Source: three-view drawing plus pictorial views. Frame: mm from the lowest corner of the part. A direction names the side the tool comes from. Coordinates: 2 decimals unless noted, no trailing zeros. Order: outer loops, then holes, each group sorted by start corner. A loop starts at its lowest first (then second) coordinate and runs counter-clockwise, first axis right, second up. Notation, with made-up numbers: (38, 13.5) -> (81, 13.5) arc R16 cw to (81, 20.5) -> close; hole circle Ø4 at (-38.5, 83.25). An arc over 180 degrees is marked (long way). One line per question, with ' | ' between items.
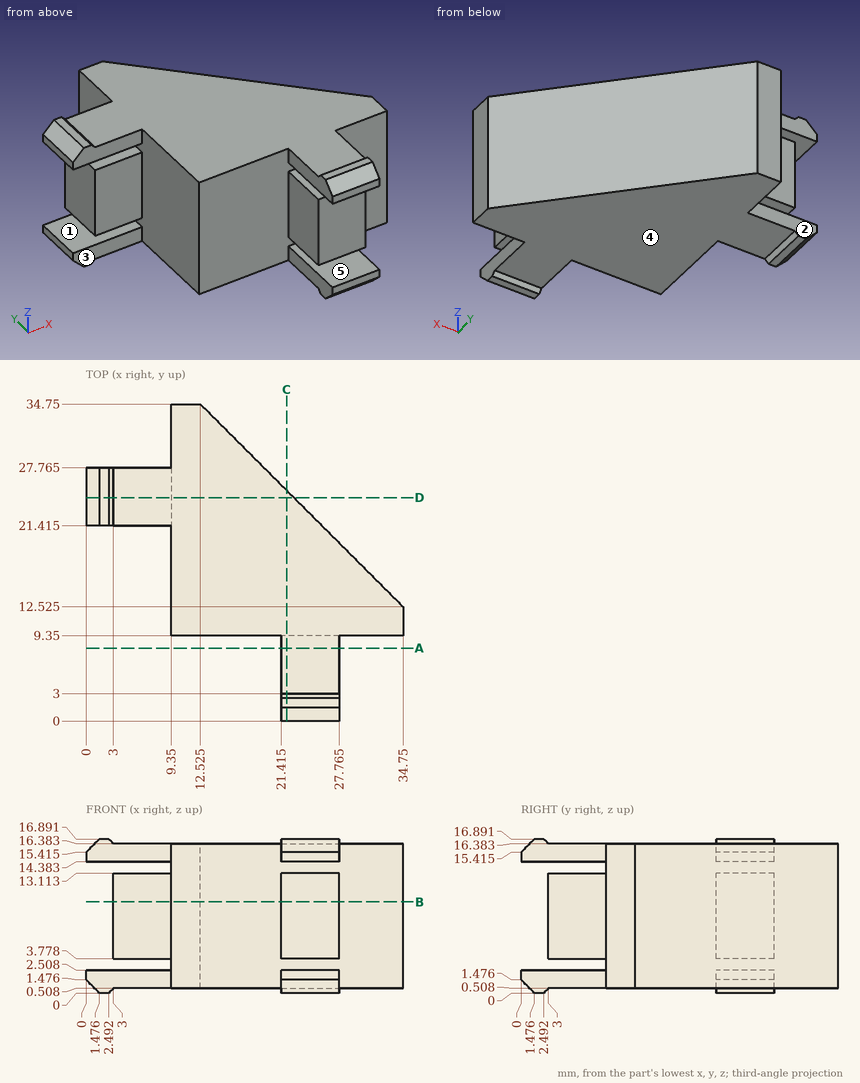
1. Access query for the marked faces 1, 2, 3, 4 and 5. Directions: +Z, -Z, +X, -X, +Y, -Y. A direction counts if a zero-diameter tool reaches every point of the face in a straight line with its end or side. Return the directions, or none.
Recorded:
face 1: -X, +Y, -Y | face 2: +Z, -Z, -X, +Y | face 3: +Z, -Z, -X, -Y | face 4: -Z, +X, +Y | face 5: +X, -X, -Y
2. Cut plane D-D, the plane y = 24.5. Return loops of the section in (x, z) (3 decimals).
Recorded:
outline: (0, 1.476) -> (1.476, 0) -> (2.492, 0) -> (3, 0.508) -> (22.775, 0.508) -> (22.775, 16.383) -> (3, 16.383) -> (2.492, 16.891) -> (1.476, 16.891) -> (0, 15.415) -> (0, 14.383) -> (9.35, 14.383) -> (9.35, 13.113) -> (3, 13.113) -> (3, 3.778) -> (9.35, 3.778) -> (9.35, 2.508) -> (0, 2.508) -> close
3. Ray query, line 1 (Z direction, x = 27.5, y = 9); line 2 (X direction, y = 11.5, z = 2.5). Return the intervals inside material, ascending. Write a range as [from, to].
Recorded:
line 1: z = [0.51, 2.51], [3.78, 13.11], [14.38, 16.38] | line 2: x = [9.35, 34.75]
4. Pin query (flat end, axial travel): pin 1 Ø3 at (x, y) = (5.5, 24) entering from +Z; pin 2 Ø8 at (y, z) = (25, 7.5) entering from -X; pin 3 Ø3 at (y, z) = (3.5, 15) entering from -X (3 decimals); pin 4 Ø12 at (x, y) = (4, 29) entering from -Z. Return the tip coordinate at first contact, or that it passes through.
Recorded:
pin 1: stops at z = 16.38 | pin 2: stops at x = 3 | pin 3: stops at x = 21.415 | pin 4: stops at z = 0
5. Cut plane A-A, the plane y = 8. Return loops of the section in (x, z) (3 decimals).
Recorded:
outline: (21.415, 0.508) -> (27.765, 0.508) -> (27.765, 2.508) -> (21.415, 2.508) -> close; (21.415, 3.778) -> (27.765, 3.778) -> (27.765, 13.113) -> (21.415, 13.113) -> close; (21.415, 14.383) -> (27.765, 14.383) -> (27.765, 16.383) -> (21.415, 16.383) -> close
6. Cut plane B-B, the plane z = 10. Return loops of the section in (x, y) (3 decimals).
Recorded:
outline: (3, 21.415) -> (9.35, 21.415) -> (9.35, 9.35) -> (21.415, 9.35) -> (21.415, 3) -> (27.765, 3) -> (27.765, 9.35) -> (34.75, 9.35) -> (34.75, 12.525) -> (12.525, 34.75) -> (9.35, 34.75) -> (9.35, 27.765) -> (3, 27.765) -> close
7. Cut plane C-C, the plane x = 22. Return loops of the section in (y, z) (3 decimals).
Recorded:
outline: (0, 1.476) -> (1.476, 0) -> (2.492, 0) -> (3, 0.508) -> (25.275, 0.508) -> (25.275, 16.383) -> (3, 16.383) -> (2.492, 16.891) -> (1.476, 16.891) -> (0, 15.415) -> (0, 14.383) -> (9.35, 14.383) -> (9.35, 13.113) -> (3, 13.113) -> (3, 3.778) -> (9.35, 3.778) -> (9.35, 2.508) -> (0, 2.508) -> close
